Here's how the part is built. I have some questions about the finished solid (model axes, mm). Face numbers are marked on the shaded views. A direction names the side the tool comes from. Coordinates: 2 decimals unless noted, no trailing zeros. Order: outer loops, then holes, each group sorted by start corner. A loop starts at its lowest first (then second) coordinate and runs counter-clockwise, first axis right, second up. Notation, with made-up numbers: (-18, -35.5) - (7, -35.5) arc R24 cw to (7, -23.5) - close; hole circle Ø6 at (-7, 38.25). An arc over 180 degrees is marked (long way). Answer as CSV lines item,"result". Start each with the question number.
Q1. Suppose I cut it at B-B (x = 38.1). Please give me the cut outline in (y, z), then the cut area to 3 significant figures.
Q2. I need wall thicknesses on line 1 (Z direction, x = 0, y = 2); line 2 (Y direction, x = 36.5, z = 3); line 3 (Y direction, x = 7, z = -20). Which ranges of each line are inside material? Lowest first, please.
Q3. For the marked faces 1, 2, 3, 4 and 5, which set-ups out of +Z, -Z, +X, -X, +Y, -Y let a thin tool reach every point of the face, with its end or its side?
Q4. Suppose I cut it at C-C (z = -38.1). Please give me the cut outline in (x, y), then the cut area to 3 significant figures.
Q5. Thinking about a two-plate mould opening in X: for the marked faces 6, 7, 8 and 9, which applies, released by +X, released by -X, zero draft, split by the parting line, or undercut?
Q6. Suppose I cut it at D-D (y = 11). Please give me the cut outline in (x, z), then the cut area to 3 significant figures.
Q7. For pin 1 Ø3 at (x, z) = (0, -38.1) entering from +Y; pin 2 Ø1 at (y, z) = (102.5, 2.5) entering from +X; pin 3 Ø3 at (y, z) = (59.5, 19) entering from +X; pin 4 Ø12 at (x, y) = (6.5, 36.5) entering from -Z, each with a flat end and sliding along its axis, tell me the tip position at first contact or that it passes through.
from build123d import *

# Parameters (mm, degrees)
SKETCH4_W                  = 12.7
SKETCH4_H                  = 2.54
F_3_0_213_DIAMETER_HOLE3_D = 5.4102


with BuildPart() as part:
    # Sketch1 → Chamber (revolve)
    with BuildSketch(Plane(origin=(0, 0, 0), x_dir=(0, 0, -1), z_dir=(1, 0, 0))):
        Polygon((31.75, 6.35), (31.75, 114.3), (44.45, 114.3), (44.45, 120.65), (31.75, 120.65), (25.4, 120.65), (25.4, 114.3), (25.4, 6.35), (25.4, 0), (31.75, 0), (44.45, 0), (44.45, 6.35), align=None)
    revolve(axis=Axis((0, 0, 0), (0, 1, 0)))

    # Sketch4 → Turbulence Rings (revolve)
    with BuildSketch(Plane(origin=(0, 0, 0), x_dir=(0, 0, -1), z_dir=(1, 0, 0))):
        with Locations((19.05, 102.87)):
            Rectangle(SKETCH4_W, SKETCH4_H)
        with Locations((19.05, 17.78)):
            Rectangle(SKETCH4_W, SKETCH4_H)
    revolve(axis=Axis((0, 0, 0), (0, 1, 0)))

    # #3 (0.213) Diameter Hole3 (through all)
    with Locations(Plane(origin=(0, 120.65, 0), x_dir=(1, 0, 0), z_dir=(0, 1, 0))):
        with Locations((0, 0), (-38.1, 0), (-32.995567884, 19.05), (-19.05, 32.995567884), (0, 38.1), (19.05, 32.995567884), (32.995567884, 19.05), (38.1, 0), (32.995567884, -19.05), (19.05, -32.995567884), (0, -38.1), (-19.05, -32.995567884), (-32.995567884, -19.05)):
            Hole(F_3_0_213_DIAMETER_HOLE3_D / 2)


solid = part.part
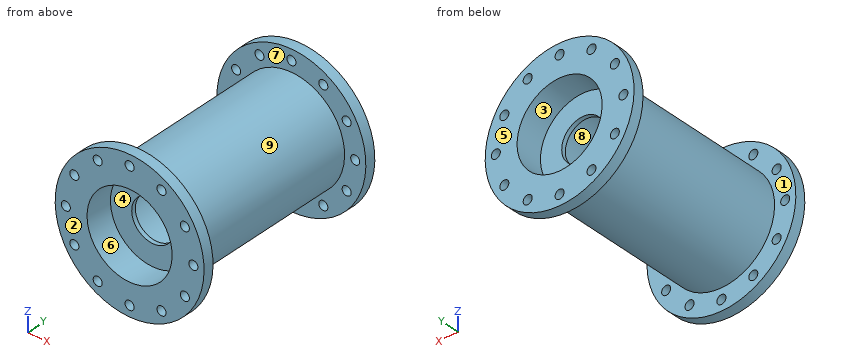
Here are the results:
1,outline,"(0, -22.9) - (6.35, -22.9) - (6.35, -2.71) - (0, -2.71) - close; (0, 2.71) - (6.35, 2.71) - (6.35, 22.9) - (0, 22.9) - close; (114.3, -22.9) - (120.65, -22.9) - (120.65, -2.71) - (114.3, -2.71) - close; (114.3, 2.71) - (120.65, 2.71) - (120.65, 22.9) - (114.3, 22.9) - close"
1,area,"513 mm²"
2,line 1,"z = -44.45 to -40.81, -35.39 to -25.4, 25.4 to 35.39, 40.81 to 44.45"
2,line 2,"y = 0 to 6.35, 114.3 to 120.65"
2,line 3,"y = 16.51 to 19.05, 101.6 to 104.14"
3,face 1,"none"
3,face 2,"+Z, -Z, +X, -X, -Y"
3,face 3,"+Y"
3,face 4,"-Y"
3,face 5,"+Z, -Z, +X, -X, +Y"
4,outline,"(-22.9, 0) - (-2.71, 0) - (-2.71, 6.35) - (-22.9, 6.35) - close; (-22.9, 114.3) - (-2.71, 114.3) - (-2.71, 120.65) - (-22.9, 120.65) - close; (2.71, 0) - (22.9, 0) - (22.9, 6.35) - (2.71, 6.35) - close; (2.71, 114.3) - (22.9, 114.3) - (22.9, 120.65) - (2.71, 120.65) - close"
4,area,"513 mm²"
5,face 6,"undercut"
5,face 7,"zero draft"
5,face 8,"undercut"
5,face 9,"split by the parting line"
6,outline,"circle Ø63.5 at (0, 0); hole circle Ø50.8 at (0, 0)"
6,area,"1,140 mm²"
7,pin 1,"passes through"
7,pin 2,"stops at x = 31.69"
7,pin 3,"stops at x = 26.49"
7,pin 4,"stops at z = -31.75"
